The model under review builds one solid part; all positions refer to its coordinate system, in mm. A direction names the side the tool comes from. Give positions to 0.01 mm unless a question says otherwise; leave off trailing zeros. Loops run counter-clockwise (first coordinate to the right, second up) from the corner with the lowest first, then second, coordinate; pieces in that order, holes last. Notation, with made-up numbers: (11, 46.5) - (33, 46.5) arc R23 ccw to (33, 60.5) - close; hole circle Ø7 at (36.5, 10). An arc over 180 degrees is marked (long way). Return JSON: item names as keys, results as strings. Group by question number.
Autodesk Fusion 360 part; units mm, degrees
sketch "Sketch1" plane through (0, 0, 0) normal (0, 0, 1) x (1, 0, 0)
  line L0 (-30, 70) -> (-30, -10)
  line L1 (70, -30) -> (-10, -30)
  line L2 (0, 70) -> (-30, 70)
  line L3 (70, 0) -> (70, -30)
  line L4 (-10, -30) -> (-30, -10)
  line L5 (5, -15) -> (-15, 5)
  line L6 (-15, 5) -> (0, 20)
  line L7 (5, -15) -> (20, 0)
  line L8 (0, 70) -> (0, 0)
  line L9 (0, 0) -> (70, 0)
  line L10 (62.5, -7) -> (27.5, -7)
  line L11 (27.5, -7) -> (27.5, -23)
  line L12 (27.5, -23) -> (62.5, -23)
  line L13 (62.5, -23) -> (62.5, -7)
  line L14 (62.5, -7) -> (27.5, -23) construction
  line L15 (27.5, -7) -> (62.5, -23) construction
  line L16 (-7, 62.5) -> (-23, 62.5)
  line L17 (-23, 62.5) -> (-23, 27.5)
  line L18 (-23, 27.5) -> (-7, 27.5)
  line L19 (-7, 27.5) -> (-7, 62.5)
  line L20 (-7, 62.5) -> (-23, 27.5) construction
  line L21 (-23, 62.5) -> (-7, 27.5) construction
  line L22 (-25, 10) -> (-15, 10)
  line L23 (-15, 10) -> (-15, 20)
  line L24 (-15, 20) -> (-25, 20)
  line L25 (-25, 20) -> (-25, 10)
  line L26 (-25, 10) -> (-15, 20) construction
  line L27 (-15, 10) -> (-25, 20) construction
  line L28 (10, -25) -> (20, -25)
  line L29 (20, -25) -> (20, -15)
  line L30 (20, -15) -> (10, -15)
  line L31 (10, -15) -> (10, -25)
  line L32 (10, -25) -> (20, -15) construction
  line L33 (20, -25) -> (10, -15) construction
  point P0 (45, -15)
  point P1 (-15, 45)
  point P2 (-20, 15)
  point P3 (15, -20)
  dimension "d15" = 35
  dimension "d16" = 16
  dimension "d17" = 16
  dimension "d18" = 35
extrude "Extrude1" add sketch "Sketch1" along normal blind 20 contours L0 L1 L2 L3 L4 L5 L6 L7 L8 L9
chamfer "Chamfer1" distance 10 angle 45 2 edges at (-15, 5, 10) (5, -15, 10)
chamfer "Chamfer3" distance 5 angle 45 8 edges at (-23, 62.5, 10) (-7, 62.5, 10) (-7, 27.5, 10) (-23, 27.5, 10) (27.5, -23, 10) (27.5, -7, 10) (62.5, -7, 10) (62.5, -23, 10)
chamfer "Chamfer4" distance 5 angle 45 4 edges at (-30, 70, 10) (0, 70, 10) (70, 0, 10) (70, -30, 10)
1) To check wall thickness, follow line 1 (X direction, y = 39.5, z = 4.75); line 2 (Y direction, x = -7.5, z = 17). State the ranges of each line that lie inside material, in increasing order.
2) Draft analysis for pull direction X (two halves, no side actions). For faces 1 (the face through (-3, 21, 0)), 2 (the face through (-3, 68, 10)), 3 (the face through (-15, 27.5, 10)), state which applies: +X half, -X half, draft (parallel to the pull), parting line (faces both ways), or undercut.
3) Tool access review of faces 4 (the face through (-15, 15, 10)), 5 (the face through (-20, -20, 10)), 6 (the face through (16, -4, 10)), 7 (the face through (-30, 28, 10)), 8 (the face through (0, 43, 10)): name each direction out of +Z, -Z, +X, -X, +Y, -Y from which nothing blocks a thin tool from reaching the whole face with its end or side.
4) We need section A-A, the plane x = 16. Write out the cut boundary in (y, z), plus the area to 3 significant figures.
5) We need section C-C, the plane y = -19.5. Write out the cut boundary in (x, z), plus the area to 3 significant figures.
6) We need section B-B, the plane y = 55.5. Write out the cut boundary in (x, z), plus the area to 3 significant figures.
7) For pin 1 Ø6.5 at (y, z) = (-14.5, 14.5) entering from -X; pin 2 Ø5 at (y, z) = (16, 13) entering from +X; pin 3 Ø3 at (x, z) = (-16, 7.5) entering from -Y, all flat-tipped, find the tip position at first contact; note any pin that passes through.
8) We need section D-D, the plane z = 14.25. Count the separate pieces of the cut face and the enclosed holes in it, plus the area to 3 significant figures.
Findings:
{
 "1": {"line 1": "x = -30 to -23, -7 to 0", "line 2": "y = -30 to -2.5, 12.5 to 32, 58 to 70"},
 "2": {"face 1": "draft", "face 2": "+X half", "face 3": "undercut"},
 "3": {"face 4": "+Z, -Z", "face 5": "+Z, -Z, -X, -Y", "face 6": "+Z, -Z, +Y", "face 7": "+Z, -Z, -X, +Y, -Y", "face 8": "+Z, -Z, +X, +Y"},
 "4": {"outline": "(-30, 0) - (-25, 0) - (-25, 20) - (-30, 20) - close; (-15, 0) - (-4, 0) - (-4, 20) - (-15, 20) - close", "area": "320 mm^2"},
 "5": {"outline": "(-20.5, 0) - (10, 0) - (10, 20) - (-20.5, 20) - close; (20, 0) - (29, 0) - (29, 20) - (20, 20) - close; (61, 0) - (70, 0) - (70, 20) - (61, 20) - close", "area": "970 mm^2"},
 "6": {"outline": "(-30, 0) - (-23, 0) - (-23, 20) - (-30, 20) - close; (-7, 0) - (0, 0) - (0, 20) - (-7, 20) - close", "area": "280 mm^2"},
 "7": {"pin 1": "stops at x = -28.75", "pin 2": "stops at x = -1.5", "pin 3": "stops at y = -25.5"},
 "8": {"separate pieces": "1", "enclosed holes": "4", "area": "3,330 mm^2"}
}
